CAD build for the part. Positions are in the model's coordinates, mm. Face numbers are marked on the shaded views. A direction names the side the tool comes from. Round coordinates to 2 decimals unless told otherwise and drop trailing zeros. Write each loop counter-clockwise with the first axis right and the second up, starting at its lowest first coordinate (ties: lowest second). Pieces come first, ordered by that corner, then holes. Notation, with made-up numbers: (42, 63) -> (78, 63) arc R34 cw to (78, 99) -> close; hole circle Ø2 at (18.5, -4). An arc over 180 degrees is marked (long way). Answer in a Markdown table with one row per item. Add a question column.
```python
from build123d import *

# Parameters (mm, degrees)
SKETCH1_R           = 12.614459283
BOSS_EXTRUDE1_DEPTH = 4.7625


with BuildPart() as part:
    # Sketch1 → Boss-Extrude1 (new body)
    with BuildSketch(Plane(origin=(0, 0, 0), x_dir=(0, 0, -1), z_dir=(1, 0, 0))):
        with BuildLine():
            Line((6.982856305, 40.645980292), (4.811028394, 34.67893215))
            ThreePointArc((4.811028394, 34.67893215), (2.180363954, 33.160117328), (0.227813255, 35.487076638))
            Line((0.227813255, 35.487076638), (0.227813255, 41.837076638))
            ThreePointArc((0.227813255, 41.837076638), (-1.359686745, 43.424576638), (-2.947186745, 41.837076638))
            Line((-2.947186745, 41.837076638), (-2.947186745, 35.487076638))
            ThreePointArc((-2.947186745, 35.487076638), (-4.899737444, 33.160117328), (-7.530401884, 34.67893215))
            Line((-7.530401884, 34.67893215), (-9.702229795, 40.645980292))
            ThreePointArc((-9.702229795, 40.645980292), (-11.736948808, 41.59478535), (-12.685753866, 39.560066337))
            Line((-12.685753866, 39.560066337), (-10.513925955, 33.593018195))
            ThreePointArc((-10.513925955, 33.593018195), (-11.552856482, 30.738580033), (-14.544337708, 31.266058885))
            Line((-14.544337708, 31.266058885), (-18.62603903, 36.130441099))
            ThreePointArc((-18.62603903, 36.130441099), (-20.862559913, 36.326111322), (-21.058230136, 34.089590438))
            Line((-21.058230136, 34.089590438), (-16.976528815, 29.225208224))
            ThreePointArc((-16.976528815, 29.225208224), (-16.976528815, 26.187578579), (-19.968010041, 25.660099726))
            Line((-19.968010041, 25.660099726), (-25.467271355, 28.835099726))
            ThreePointArc((-25.467271355, 28.835099726), (-27.635836683, 28.254034398), (-27.054771355, 26.085469069))
            Line((-27.054771355, 26.085469069), (-21.555510041, 22.910469069))
            ThreePointArc((-21.555510041, 22.910469069), (-20.516579514, 20.056030907), (-23.147243954, 18.537216084))
            Line((-23.147243954, 18.537216084), (-29.400773186, 19.639882012))
            ThreePointArc((-29.400773186, 19.639882012), (-31.239821976, 18.352166186), (-29.95210615, 16.513117396))
            Line((-29.95210615, 16.513117396), (-23.698576918, 15.410451468))
            ThreePointArc((-23.698576918, 15.410451468), (-21.746026219, 13.083492158), (-23.698576918, 10.756532847))
            Line((-23.698576918, 10.756532847), (-29.95210615, 9.653866919))
            ThreePointArc((-29.95210615, 9.653866919), (-31.239821976, 7.814818129), (-29.400773186, 6.527102303))
            Line((-29.400773186, 6.527102303), (-23.147243954, 7.629768232))
            ThreePointArc((-23.147243954, 7.629768232), (-20.516579514, 6.110953409), (-21.555510041, 3.256515246))
            Line((-21.555510041, 3.256515246), (-27.054771355, 0.081515246))
            ThreePointArc((-27.054771355, 0.081515246), (-27.635836683, -2.087050082), (-25.467271355, -2.668115411))
            Line((-25.467271355, -2.668115411), (-19.968010041, 0.506884589))
            ThreePointArc((-19.968010041, 0.506884589), (-16.976528815, -0.020594263), (-16.976528815, -3.058223909))
            Line((-16.976528815, -3.058223909), (-21.058230136, -7.922606123))
            ThreePointArc((-21.058230136, -7.922606123), (-20.862559913, -10.159127007), (-18.62603903, -9.963456784))
            Line((-18.62603903, -9.963456784), (-14.544337708, -5.09907457))
            ThreePointArc((-14.544337708, -5.09907457), (-11.552856482, -4.571595717), (-10.513925955, -7.42603388))
            Line((-10.513925955, -7.42603388), (-12.685753866, -13.393082022))
            ThreePointArc((-12.685753866, -13.393082022), (-11.736948808, -15.427801035), (-9.702229795, -14.478995977))
            Line((-9.702229795, -14.478995977), (-7.530401884, -8.511947835))
            ThreePointArc((-7.530401884, -8.511947835), (-4.899737444, -6.993133012), (-2.947186745, -9.320092323))
            Line((-2.947186745, -9.320092323), (-2.947186745, -15.670092323))
            ThreePointArc((-2.947186745, -15.670092323), (-1.359686745, -17.257592323), (0.227813255, -15.670092323))
            Line((0.227813255, -15.670092323), (0.227813255, -9.320092323))
            ThreePointArc((0.227813255, -9.320092323), (2.180363954, -6.993133012), (4.811028394, -8.511947835))
            Line((4.811028394, -8.511947835), (6.982856305, -14.478995977))
            ThreePointArc((6.982856305, -14.478995977), (9.017575318, -15.427801035), (9.966380376, -13.393082022))
            Line((9.966380376, -13.393082022), (7.794552465, -7.42603388))
            ThreePointArc((7.794552465, -7.42603388), (8.833482992, -4.571595717), (11.824964218, -5.09907457))
            Line((11.824964218, -5.09907457), (15.90666554, -9.963456784))
            ThreePointArc((15.90666554, -9.963456784), (18.143186423, -10.159127007), (18.338856646, -7.922606123))
            Line((18.338856646, -7.922606123), (14.257155325, -3.058223909))
            ThreePointArc((14.257155325, -3.058223909), (14.257155325, -0.020594263), (17.248636551, 0.506884589))
            Line((17.248636551, 0.506884589), (22.747897865, -2.668115411))
            ThreePointArc((22.747897865, -2.668115411), (24.916463193, -2.087050082), (24.335397865, 0.081515246))
            Line((24.335397865, 0.081515246), (18.836136551, 3.256515246))
            ThreePointArc((18.836136551, 3.256515246), (17.797206024, 6.110953409), (20.427870464, 7.629768232))
            Line((20.427870464, 7.629768232), (26.681399696, 6.527102303))
            ThreePointArc((26.681399696, 6.527102303), (28.520448486, 7.814818129), (27.23273266, 9.653866919))
            Line((27.23273266, 9.653866919), (20.979203428, 10.756532847))
            ThreePointArc((20.979203428, 10.756532847), (19.026652729, 13.083492158), (20.979203428, 15.410451468))
            Line((20.979203428, 15.410451468), (27.23273266, 16.513117396))
            ThreePointArc((27.23273266, 16.513117396), (28.520448486, 18.352166186), (26.681399696, 19.639882012))
            Line((26.681399696, 19.639882012), (20.427870464, 18.537216084))
            ThreePointArc((20.427870464, 18.537216084), (17.797206024, 20.056030907), (18.836136551, 22.910469069))
            Line((18.836136551, 22.910469069), (24.335397865, 26.085469069))
            ThreePointArc((24.335397865, 26.085469069), (24.916463193, 28.254034398), (22.747897865, 28.835099726))
            Line((22.747897865, 28.835099726), (17.248636551, 25.660099726))
            ThreePointArc((17.248636551, 25.660099726), (14.257155325, 26.187578579), (14.257155325, 29.225208224))
            Line((14.257155325, 29.225208224), (18.338856646, 34.089590438))
            ThreePointArc((18.338856646, 34.089590438), (18.143186423, 36.326111322), (15.90666554, 36.130441099))
            Line((15.90666554, 36.130441099), (11.824964218, 31.266058885))
            ThreePointArc((11.824964218, 31.266058885), (8.833482992, 30.738580033), (7.794552465, 33.593018195))
            Line((7.794552465, 33.593018195), (9.966380376, 39.560066337))
            ThreePointArc((9.966380376, 39.560066337), (9.017575318, 41.59478535), (6.982856305, 40.645980292))
        make_face()
        with Locations(Location((-1.359686745, 13.083492158, 0), (0, 0, 180))):
            Circle(SKETCH1_R, mode=Mode.SUBTRACT)
    extrude(amount=BOSS_EXTRUDE1_DEPTH)


solid = part.part
```
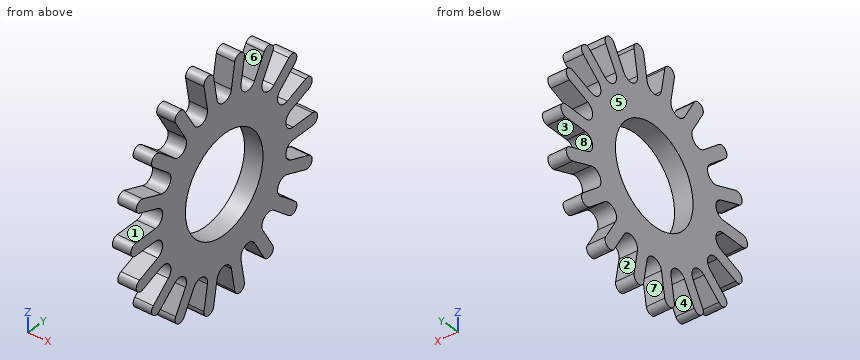
Item 1: Pin check, flat tips, straight feed: pin 1 (2 mm diameter, centred on x = 4, z = 10, fed in from -Y); pin 2 (1.4 mm diameter, centred on x = 1.5, y = -12, fed in from +Z). Stop position of each tip, or through.
Item 2: Drill centre lines: probe 1 along Z at (x, y) = (0.4, -8.5); probe 2 along Y at (x, z) = (3, -24.5); probe 3 along Z at (x, y) = (1.4, 41). Where is each one in solid material? Low to high.
Item 3: Two-plate mould, pull along Y, no slides. Class the marked faces 5, 6, 7 and 8: +Y half, -Y half, draft (parallel to the pull), parting line (faces both ways), or undercut.
Item 4: Saw through at B-B on y = 32. Give the cut face in (x, z), then the cut area to 3 significant figures.
Item 5: Tool access for the marked faces 1, 2, 3 and 4: list every direction of +Z, -Z, +X, -X, +Y, -Y with a clear straight run to the whole face (end or side of a thin tool).
Item 6: Saw through at A-A on y = 22. Give the cut face in (x, z), then the cut area to 3 significant figures.
Recorded:
| question | item | result |
|---|---|---|
| 1 | pin 1 | y = -15.51 |
| 1 | pin 2 | z = 12.43 |
| 2 | probe 1 | -18.65 to -14.68, -8.19 to -4.81, -0.37 to 3.09, 7.53 to 10.9, 17.4 to 21.37 |
| 2 | probe 2 | -2.56 to -0.03, 6.91 to 10.14, 16.03 to 19.26, 26.19 to 28.73 |
| 2 | probe 3 | -9.78 to -7.16, -0.23 to 2.95, 9.88 to 12.5 |
| 3 | face 5 | draft |
| 3 | face 6 | undercut |
| 3 | face 7 | undercut |
| 3 | face 8 | +Y half |
| 4 | outline | (0, -16.59) -> (4.76, -16.59) -> (4.76, -12.44) -> (0, -12.44) -> close; (0, -7.79) -> (4.76, -7.79) -> (4.76, 10.51) -> (0, 10.51) -> close; (0, 15.16) -> (4.76, 15.16) -> (4.76, 19.3) -> (0, 19.3) -> close |
| 4 | area | 127 mm2 |
| 5 | face 1 | +X, -X, -Y |
| 5 | face 2 | +X, -X |
| 5 | face 3 | +X, -X, +Y |
| 5 | face 4 | -Z, +X, -X |
| 6 | outline | (0, -17.95) -> (4.76, -17.95) -> (4.76, -7.56) -> (0, -7.56) -> close; (0, 10.28) -> (4.76, 10.28) -> (4.76, 20.66) -> (0, 20.66) -> close |
| 6 | area | 98.9 mm2 |
